Geometry check sheet. Reference: drawing and pictorial views, mm from the part's lowest x, y, z. Give positions to 0.01 mm unless a question says otherwise; leave off trailing zeros. Order: outer loops, then holes, each group sorted by start corner. A loop starts at its lowest first (then second) coordinate and runs counter-clockwise, first axis right, second up. Notation, with made-up numbers: (88, 31.5) - (124, 31.5) arc R14 cw to (124, 39.5) - close; hole circle Ø11 at (37, 36.5). An arc over 180 degrees is marked (long way). Answer as a JSON object with one key per item and string values.
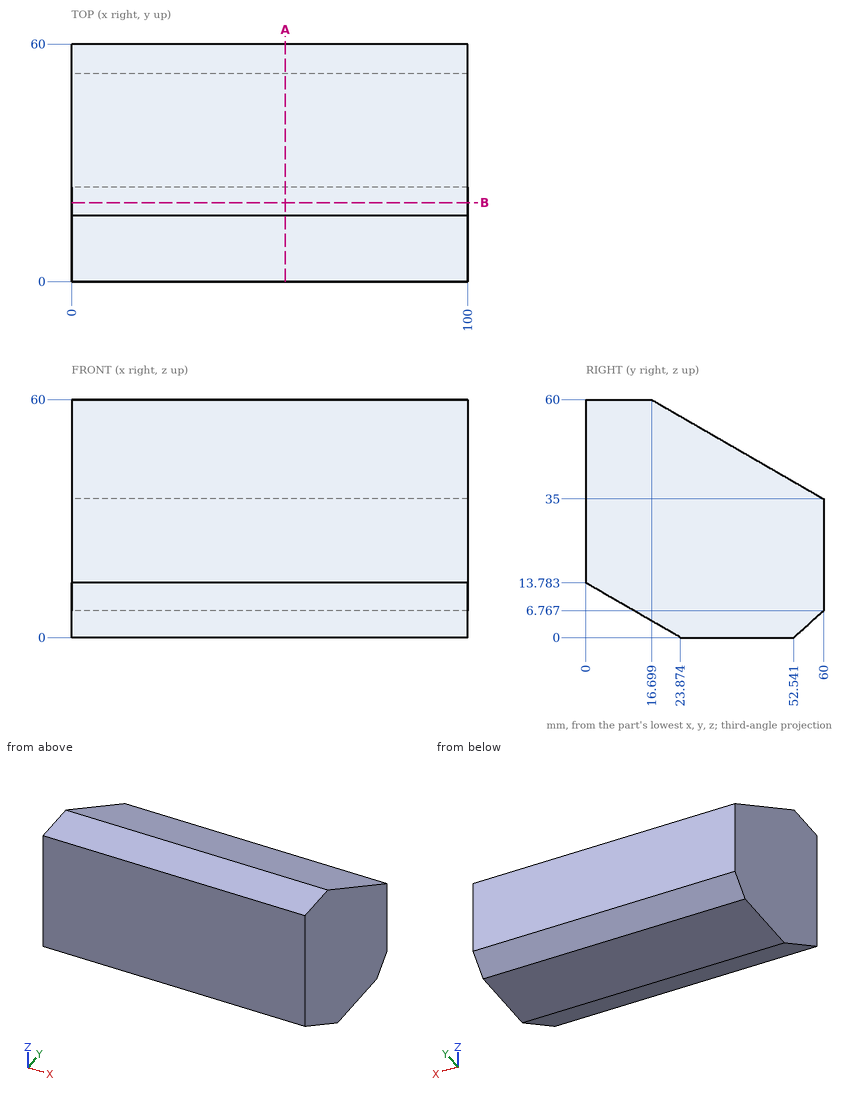
(1) Material ranges on line 1 along Z through (x, y) = (82, 42); line 2 along Z through (x, y) = (93, 51.5), recorded low to high. Write a range as [from, to].
Computed values:
{"line 1": "z = [0, 45.39]", "line 2": "z = [0, 39.91]"}
(2) Gauge pin test, flat ends, axial feed: pin 1 Ø1 at (x, z) = (35, 18.5) entering from -Y; pin 2 Ø6 at (x, y) = (76.5, 18) entering from -Z; pin 3 Ø4 at (x, y) = (44.5, 21.5) entering from +Z; pin 4 Ø1 at (x, y) = (22, 25.5) entering from +Z. Record the tip position at first contact, or that the pin passes through.
Computed values:
{"pin 1": "stops at y = 0", "pin 2": "stops at z = 1.66", "pin 3": "stops at z = 58.38", "pin 4": "stops at z = 55.21"}
(3) Section check B-B (y = 20). Record the cut outline in (x, z).
Computed values:
{"outline": "(0, 2.24) - (100, 2.24) - (100, 58.09) - (0, 58.09) - close"}
(4) Section check A-A (x = 54). Record the cut outline in (y, z), then the cut area to 3 significant figures.
Computed values:
{"outline": "(0, 13.78) - (23.87, 0) - (52.54, 0) - (60, 6.77) - (60, 35) - (16.7, 60) - (0, 60) - close", "area": "2,870 mm²"}
